Can you work these out from the model? Positions are in its coordinate system, mm. A direction names the side the tool comes from. Coordinates: 2 decimals unless noted, no trailing zeros. Loops run counter-clockwise (first coordinate to the right, second up) from the corner with the lowest first, then second, coordinate; pieces in that order, holes last. Notation, with made-up numbers: (61.5, -18.5) - (115.5, -18.5) arc R14 ccw to (115.5, -10.5) - close; hole circle Ø8 at (-11, 7). An arc over 180 degrees is marked (long way). Put each result on its own line as item: value. Start each with the question number.
from build123d import *

# Parameters (mm, degrees)
SKETCH1_W           = 133
SKETCH1_H           = 110
BOSS_EXTRUDE1_DEPTH = 3
SKETCH2_W           = 50
SKETCH2_H           = 18
BOSS_EXTRUDE2_DEPTH = 3
SKETCH3_W           = 125
SKETCH3_H           = 15
BOSS_EXTRUDE3_DEPTH = 3
SKETCH4_R           = 15.25
CUT_EXTRUDE1_DEPTH  = 3
SKETCH5_R           = 16.375
CUT_EXTRUDE2_DEPTH  = 1


with BuildPart() as part:
    # Sketch1 → Boss-Extrude1 (new body)
    with BuildSketch(Plane(origin=(0, 0, 0), x_dir=(1, 0, 0), z_dir=(0, 1, 0))):
        with Locations((66.5, 55)):
            Rectangle(SKETCH1_W, SKETCH1_H)
    extrude(amount=BOSS_EXTRUDE1_DEPTH)

    # Sketch2 → Boss-Extrude2 (add)
    with BuildSketch(Plane(origin=(0, 3, 0), x_dir=(1, 0, 0), z_dir=(0, 1, 0))):
        with Locations((25, 109)):
            Rectangle(SKETCH2_W, SKETCH2_H)
    extrude(amount=BOSS_EXTRUDE2_DEPTH)

    # Sketch3 → Boss-Extrude3 (add)
    with BuildSketch(Plane(origin=(0, 3, 0), x_dir=(1, 0, 0), z_dir=(0, 1, 0))):
        with Locations((70.5, 2.5)):
            Rectangle(SKETCH3_W, SKETCH3_H)
    extrude(amount=BOSS_EXTRUDE3_DEPTH)

    # Sketch4 → Cut-Extrude1 (cut)
    with BuildSketch(Plane.XZ):
        with Locations((25.5, -81.25)):
            Circle(SKETCH4_R)
        with Locations((32.5, -42.75)):
            Circle(SKETCH4_R)
        with Locations((61.5, -81.25)):
            Circle(SKETCH4_R)
        with Locations((97.5, -81.25)):
            Circle(SKETCH4_R)
        with Locations((130.5, -67.25)):
            Circle(SKETCH4_R)
        with Locations((68.5, -42.75)):
            Circle(SKETCH4_R)
        with Locations((104.5, -42.75)):
            Circle(SKETCH4_R)
        with Locations((137.5, -28.75)):
            Circle(SKETCH4_R)
    extrude(amount=-CUT_EXTRUDE1_DEPTH, mode=Mode.SUBTRACT)

    # Sketch5 → Cut-Extrude2 (cut)
    with BuildSketch(Plane(origin=(0, 3, 0), x_dir=(1, 0, 0), z_dir=(0, 1, 0))):
        with Locations((25.5, 81.25)):
            Circle(SKETCH5_R)
        with Locations((61.5, 81.25)):
            Circle(SKETCH5_R)
        with Locations((97.5, 81.25)):
            Circle(SKETCH5_R)
        with Locations((32.5, 42.75)):
            Circle(SKETCH5_R)
        with Locations((68.5, 42.75)):
            Circle(SKETCH5_R)
        with Locations((104.5, 42.75)):
            Circle(SKETCH5_R)
        with Locations((130.5, 67.25)):
            Circle(SKETCH5_R)
        with Locations((137.5, 28.75)):
            Circle(SKETCH5_R)
    extrude(amount=-CUT_EXTRUDE2_DEPTH, mode=Mode.SUBTRACT)


solid = part.part
Q1. I want a section at C-C on x = 61.5. List the corners of the cut face in (y, z) for me (3 decimals), and give its area (3 significant figures).
Q2. I want a section at B-B on z = -108. List the corners of the cut face in (x, y) for me, and give its area (3 significant figures).
Q3. I want a section at A-A on x = 32.5. List the corners of the cut face in (y, z) for me (3 decimals).
Q4. On a 3-axis mill with a long thin cutter (end or side, diameter ignored), from which of +Z, -Z, +X, -X, +Y, -Y can I reach the whole of each face in a straight line? I mean faces 1 (the flat face through (66, 1, -110)), 2 (the flat face through (70, 4, -10)), 3 (the flat face through (64, 2, -28)), 4 (the flat face through (70, 3, 2)), 5 (the cylindrical face through (121.128, 2.507, -29.046)). Say none if no direction works.
Q5. Please list where these lines run through material, in increasing order: line 1 along Z through (x, y) = (32.5, 2.2) (3 decimals); line 2 along Z through (x, y) = (130.5, 1.6); line 3 along Z through (x, y) = (85, 5.7). Write a range as [from, to].
Q6. Will these pins go through, and if not, where does the flat tip stop? pin 1 (0.9 mm diameter, centred on y = 4, z = -2.5, fed in from -X); pin 2 (1.5 mm diameter, centred on x = 79.5, y = 1.5, fed in from +Z); pin 3 (1.5 mm diameter, centred on y = 5, z = -60, fed in from +X); pin 4 (2.5 mm diameter, centred on x = 29, z = -115.5, fed in from -Y).
Calculated:
1. outline: (0, -110) - (3, -110) - (3, -97.625) - (2, -97.625) - (2, -96.5) - (0, -96.5) - close; (0, -66) - (2, -66) - (2, -64.875) - (3, -64.875) - (3, -57.553) - (2, -57.553) - (2, -56.299) - (0, -56.299) - close; (0, -29.201) - (2, -29.201) - (2, -27.947) - (3, -27.947) - (3, -10) - (6, -10) - (6, 5) - (3, 5) - (3, 0) - (0, 0) - close
1. area: 197 mm2
2. outline: (0, 0) - (133, 0) - (133, 3) - (50, 3) - (50, 6) - (0, 6) - close
2. area: 549 mm2
3. outline: (0, -110) - (3, -110) - (3, -118) - (6, -118) - (6, -100) - (3, -100) - (3, -96.053) - (2, -96.053) - (2, -94.799) - (0, -94.799) - close; (0, -67.701) - (2, -67.701) - (2, -66.447) - (3, -66.447) - (3, -59.125) - (2, -59.125) - (2, -58) - (0, -58) - close; (0, -27.5) - (2, -27.5) - (2, -26.375) - (3, -26.375) - (3, -10) - (6, -10) - (6, 5) - (3, 5) - (3, 0) - (0, 0) - close
4. face 1: -Z, +X, -X, -Y
4. face 2: +X, -X, +Y
4. face 3: +Y
4. face 4: +Z, +X, -X, -Y
4. face 5: +X, +Y
5. line 1: [-110, -96.053], [-66.447, -59.125], [-26.375, 0]
5. line 2: [-110, -82.5], [-52, -42.3], [-15.2, 0]
5. line 3: [-10, 5]
6. pin 1: x = 8
6. pin 2: z = 0
6. pin 3: through
6. pin 4: y = 3
